from build123d import *

# Parameters (mm, degrees)
F0_R     = 37.5
F0_R_2   = 35
F1_DEPTH = 30
F2_R     = 36.5
F2_R_2   = 35
F3_DEPTH = 1
F4_R     = 39
F4_R_2   = 36.5
F5_DEPTH = 5
F6_SIZE2 = 3
F6_SIZE  = 25
F7_SIZE  = 5


with BuildPart() as f1:
    # F0 (on Top) → F1 (new body)
    with BuildSketch(Plane.XY):
        Circle(F0_R)
        Circle(F0_R_2, mode=Mode.SUBTRACT)
    extrude(amount=F1_DEPTH)

    # F2 (on face) → F3 (join)
    with BuildSketch(Plane.XY.offset(30)):
        Circle(F2_R)
        Circle(F2_R_2, mode=Mode.SUBTRACT)
        Circle(F2_R_2)
    extrude(amount=F3_DEPTH)

    # F4 (on face) → F5 (join)
    with BuildSketch(Plane.XY.offset(31)):
        Circle(F4_R)
        Circle(F4_R_2, mode=Mode.SUBTRACT)
        Circle(F4_R_2)
    extrude(amount=F5_DEPTH)

    # F6
    f6_edges = [f1.edges().sort_by_distance(p)[0] for p in [
        (-39, 0, 36),
    ]]
    f6_side = f1.faces().sort_by_distance((0, 0, 36))[0]
    chamfer(f6_edges, length=F6_SIZE, length2=F6_SIZE2, reference=f6_side)

    # F7
    f7_edges = [f1.edges().sort_by_distance(p)[0] for p in [
        (-14, 0, 36),
    ]]
    chamfer(f7_edges, length=F7_SIZE)


solid = f1.part
The model under review builds one solid part; all positions refer to its coordinate system, in mm. A direction names the side the tool comes from. Round coordinates to 2 decimals unless told otherwise and drop trailing zeros. Order: outer loops, then holes, each group sorted by start corner. A loop starts at its lowest first (then second) coordinate and runs counter-clockwise, first axis right, second up. Notation, with made-up numbers: (31, 13) -> (74, 13) arc R18 cw to (74, 34) -> close; hole circle Ø1 at (-23, 8.25). An arc over 180 degrees is marked (long way). Use CSV: the item, a comma, the result in double quotes. Start each with the question number.
(1) Tool access review of faces 5 (the face through (8, -36, 30)), 6 (the face through (-4.383, -19.737, 35.254)), 7 (the face through (-28, -21, 15)): name each direction out of +Z, -Z, +X, -X, +Y, -Y from which nothing blocks a thin tool from reaching the whole face with its end or side.
(2) Mouldability with a two-part tool opening along Z and no side actions: class faces 1 (the face through (-7.912, -35.632, 30.493)), 2 (the face through (-5.077, 38.668, 31.986)), 3 (the face through (9.05, 2.85, 35.97)), 4 (the face through (26, -26, 31)) as pulls with the +Z half, pulls with the -Z half, needs draft (parallel to the pull), parting line crosses it, or undercut.
(3) Consider section D-D on z = 34. Write out the cut boundary in (x, y).
(4) Consider section C-C on z = 26. Write out the cut boundary in (x, y).
(5) Insertion check: pin 1 (3 mm diameter, centred on x = 18, y = 13.5, fed in from +Z); pin 2 (5 mm diameter, centred on x = 24, y = -12, fed in from +Z); pin 3 (12 mm diameter, centred on x = 5, z = 8, fed in from -Y). Each pin has a flat end and moves straight along its axis. Give the tip position at first contact, or say it passes through.
(6) Wall thickness on probe 1 along Y at (x, z) = (-0.5, 26); probe 2 along Z at (x, y) = (13.5, 34.5); probe 3 along X at (y, z) = (5, 10): over which ranges is each line inside the solid? List them lowest first. Write a range as from..to.
(7) Consider section A-A on x = 0. Write out the cut boundary in (y, z), and give its area (3 significant figures).
Responses:
1,face 5,"none"
1,face 6,"+Z"
1,face 7,"-Z"
2,face 1,"undercut"
2,face 2,"needs draft"
2,face 3,"pulls with the +Z half"
2,face 4,"undercut"
3,outline,"circle Ø61.33 at (0, 0)"
4,outline,"circle Ø75 at (0, 0); hole circle Ø70 at (0, 0)"
5,pin 1,"z = 35.16"
5,pin 2,"z = 34.76"
5,pin 3,"y = -37.5"
6,probe 1,"-37.5..-35, 35..37.5"
6,probe 2,"0..30, 31..33.23"
6,probe 3,"-37.17..-34.64, 34.64..37.17"
7,outline,"(-39, 31) -> (-36.5, 31) -> (-36.5, 30) -> (-37.5, 30) -> (-37.5, 0) -> (-35, 0) -> (-35, 30) -> (35, 30) -> (35, 0) -> (37.5, 0) -> (37.5, 30) -> (36.5, 30) -> (36.5, 31) -> (39, 31) -> (39, 33) -> (18.96, 35.4) -> (9, 36) -> (-9, 36) -> (-18.96, 35.4) -> (-39, 33) -> close"
7,area,"535 mm²"
